For this review, take the finished solid that the model builds, in its own axes (mm). A direction names the side the tool comes from. Round coordinates to 2 decimals unless told otherwise and drop trailing zeros. Order: outer loops, then holes, each group sorted by start corner. A loop starts at its lowest first (then second) coordinate and runs counter-clockwise, first axis right, second up. Notation, with made-up numbers: M -14.75,82 L 38.25,82 A11 cw 38.25,89 Z; hole C 69.5,36 d9. An arc over 180 degrees is marked long. Use a Markdown table: item, result.
from build123d import *

# Parameters (mm, degrees)
SKETCH1_R           = 25.4
BOSS_EXTRUDE1_DEPTH = 15
BOSS_EXTRUDE2_DEPTH = 25


with BuildPart() as part:
    # Sketch1 → Boss-Extrude1 (new body)
    # profile 1 of 2: a face of its own
    with BuildSketch(Plane(origin=(0, 0, 0), x_dir=(1, 0, 0), z_dir=(0, 1, 0))):
        with Locations(Location((0, 0, 0), (0, 0, 270))):
            Circle(SKETCH1_R)
        Polygon((12.958072873, 7.555683121), (-0.064377089, 14.999861852), (-13.022449962, 7.444178731), (-12.958072873, -7.555683121), (0.064377089, -14.999861852), (13.022449962, -7.444178731), align=None, mode=Mode.SUBTRACT)
    # profile 2 of 2: a face of its own
    with BuildSketch(Plane(origin=(0, 0, 0), x_dir=(1, 0, 0), z_dir=(0, 1, 0))):
        Polygon((13.022449962, -7.444178731), (12.958072873, 7.555683121), (-0.064377089, 14.999861852), (-13.022449962, 7.444178731), (-12.958072873, -7.555683121), (0.064377089, -14.999861852), align=None)
    extrude(amount=-BOSS_EXTRUDE1_DEPTH)

    # Sketch1_3 → Boss-Extrude2 (add)
    with BuildSketch(Plane(origin=(0, 0, 0), x_dir=(1, 0, 0), z_dir=(0, 1, 0))):
        Polygon((13.022449962, -7.444178731), (12.958072873, 7.555683121), (-0.064377089, 14.999861852), (-13.022449962, 7.444178731), (-12.958072873, -7.555683121), (0.064377089, -14.999861852), align=None)
    extrude(amount=BOSS_EXTRUDE2_DEPTH)


solid = part.part
Q1. Add section B-B (x = -2.5). Write out the cut boundary in (y, z).
Determined:
| item | result |
|---|---|
| outline | M -15,-25.28 L 0,-25.28 L 0,-13.58 L 25,-13.58 L 25,13.53 L 0,13.53 L 0,25.28 L -15,25.28 Z |
Q2. Wall thickness on line 1 along Y through (x, z) = (-21, 9.5); line 2 along Z through (x, y) = (-14, -1.5); line 3 along X through (y, z) = (1, -4.5): over which ranges is each line inside the solid? List them lowest first. Write a range as [from, to].
Determined:
| item | result |
|---|---|
| line 1 | y = [-15, 0] |
| line 2 | z = [-21.19, 21.19] |
| line 3 | x = [-13.01, 12.97] |
Q3. Clearance check with flat-ended pins moving along their axes: pin 1 (5 mm diameter, centred on y = -4.5, z = -4.5, fed in from -X); pin 2 (1 mm diameter, centred on x = 11, y = 12.5, fed in from +Z) (3 decimals); pin 3 (5 mm diameter, centred on y = -10, z = -2.5, fed in from +X). State where each tip first meets the part, or that it passes through.
Determined:
| item | result |
|---|---|
| pin 1 | stops at x = -25.32 |
| pin 2 | stops at z = 8.915 |
| pin 3 | stops at x = 25.4 |
Q4. Machinability: for faces 1 (the flat face through (-6, 0, -12)), 2 (the flat face through (-6.453, 12.325, -11.275)), 3 (the flat face through (-6.538, 12.325, 11.226)), 4 (the flat face through (6.538, 12.325, -11.226)), 5 (the flat face through (6.453, 12.325, 11.275)), which of the approach directions +Z, -Z, +X, -X, +Y, -Y give a long, thin tool a straight path to every point of the face, cutting with its end or side? Answer none if there is none.
Determined:
| item | result |
|---|---|
| face 1 | +Y |
| face 2 | -Z, -X, +Y |
| face 3 | +Z, -X, +Y |
| face 4 | -Z, +X, +Y |
| face 5 | +Z, +X, +Y |
Q5. Add section D-D (x = 17.5). Write out the cut boundary in (y, z), then the cut area to 3 significant figures.
Determined:
| item | result |
|---|---|
| outline | M -15,-18.41 L 0,-18.41 L 0,18.41 L -15,18.41 Z |
| area | 552 mm^2 |
Q6. Add section C-C (z = -13.5). Write out the cut boundary in (x, y), then the cut area to 3 significant figures.
Determined:
| item | result |
|---|---|
| outline | M -21.52,-15 L 21.52,-15 L 21.52,0 L 2.56,0 L 2.56,25 L -2.64,25 L -2.64,0 L -21.52,0 Z |
| area | 775 mm^2 |
Q7. Add section A-A (y = 10.5). Write out the cut boundary in (x, z), then the cut area to 3 significant figures.
Determined:
| item | result |
|---|---|
| outline | M -13.02,-7.44 L -0.06,-15 L 12.96,-7.56 L 13.02,7.44 L 0.06,15 L -12.96,7.56 Z |
| area | 585 mm^2 |
